The drawing under review shows one solid part. Ordinate dimensions are in mm from its lowest x, y, z. A direction names the side the tool comes from. Round coordinates to 2 decimals unless told otherwise and drop trailing zeros. Order: outer loops, then holes, each group sorted by start corner. A loop starts at its lowest first (then second) coordinate and runs counter-clockwise, first axis right, second up. Notation, with made-up numbers: M 27,-22.75 L 83,-22.75 A21 cw 83,15.25 Z; hole C -13,79 d3. An arc over 180 degrees is marked long. Answer as a JSON object with one key per item and string values.
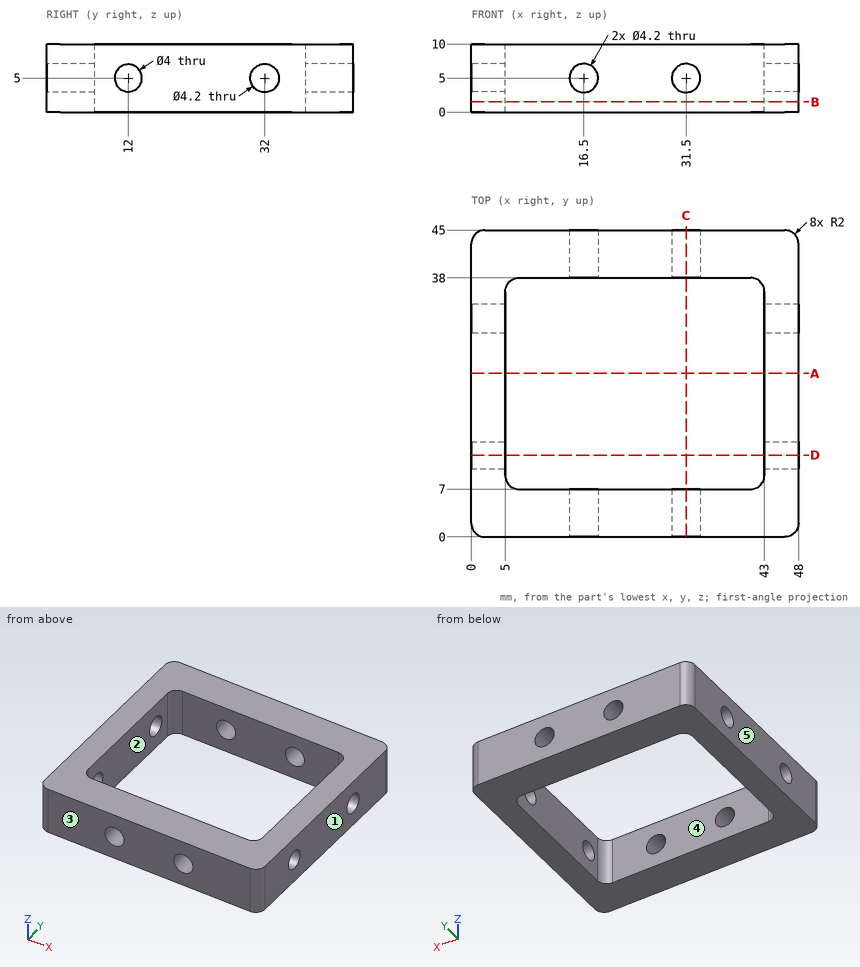
1) Add section B-B on z = 1.5. State the section outline as (x, y) points.
Geometry check:
{"outline": "M 0,2 A2 ccw 2,0 L 46,0 A2 ccw 48,2 L 48,43 A2 ccw 46,45 L 2,45 A2 ccw 0,43 Z; hole M 5,9 A2 ccw 7,7 L 41,7 A2 ccw 43,9 L 43,36 A2 ccw 41,38 L 7,38 A2 ccw 5,36 Z"}
2) Add section D-D on y = 12. State the section outline as (x, z) points.
Geometry check:
{"outline": "M 0,0 L 5,0 L 5,3 L 0,3 Z; M 0,7 L 5,7 L 5,10 L 0,10 Z; M 43,0 L 48,0 L 48,3 L 43,3 Z; M 43,7 L 48,7 L 48,10 L 43,10 Z"}
3) For L1, parallel to Y at x = 44.7, z = 5; L2, parallel to Z at x = 31.5, y = 41.25; L3, parallel to X at y = 25.5, z = 2, list the stretches that pass through material, from the lowest coordinate up.
Geometry check:
{"L1": "y = 0 to 10, 14 to 29.9, 34.1 to 45", "L2": "z = 0 to 2.9, 7.1 to 10", "L3": "x = 0 to 5, 43 to 48"}
4) Mouldability with a two-part tool opening along Y and no side actions: class the marked faces 3, 4 and 5 as +Y half, -Y half, draft (parallel to the pull), parting line (faces both ways), or undercut.
Geometry check:
{"face 3": "-Y half", "face 4": "undercut", "face 5": "draft"}
5) Insertion check: P1, Ø4, axis at y = 32, z = 5, coming from the -X side (3 decimals). The pin has a flat end and moves straight along its axis. Give the tip position at first contact, or say it passes through.
Geometry check:
{"P1": "passes through"}
6) Add section C-C on x = 31.5. State the section outline as (y, z) points, and give its area (3 significant figures).
Geometry check:
{"outline": "M 0,0 L 7,0 L 7,2.9 L 0,2.9 Z; M 0,7.1 L 7,7.1 L 7,10 L 0,10 Z; M 38,0 L 45,0 L 45,2.9 L 38,2.9 Z; M 38,7.1 L 45,7.1 L 45,10 L 38,10 Z", "area": "81.2 mm²"}
7) Add section A-A on y = 24. State the section outline as (x, z) points.
Geometry check:
{"outline": "M 0,0 L 5,0 L 5,10 L 0,10 Z; M 43,0 L 48,0 L 48,10 L 43,10 Z"}
8) Machinability: for the marked faces 1 and 2, which of the approach directions +Z, -Z, +X, -X, +Y, -Y give a long, thin tool a straight path to every point of the face, cutting with its end or side? Answer none if there is none.
Geometry check:
{"face 1": "+Z, -Z, +X, +Y, -Y", "face 2": "+Z, -Z"}
